Read the model definition and answer for the solid it produces. Units are mm, in the model's axes. A direction names the side the tool comes from. Give positions to 0.01 mm unless a question says otherwise; leave off trailing zeros. Write each loop counter-clockwise with the first axis right and the second up, starting at its lowest first coordinate (ties: lowest second). Pieces come first, ordered by that corner, then holes. Notation, with made-up numbers: (21.25, 79.5) - (31.25, 79.5) arc R30 cw to (31.25, 114.5) - close; hole circle Ø10 at (10, 86). An arc over 180 degrees is marked (long way). Answer as a JSON object with one key per item and string values. Group by question number.
```python
from build123d import *

# Parameters (mm, degrees)
SKETCH1_W           = 95
SKETCH1_H           = 50
BOSS_EXTRUDE1_DEPTH = 5
SKETCH2_W           = 14.5
SKETCH2_H           = 6
BOSS_EXTRUDE2_DEPTH = 32
SKETCH4_R           = 2.75
CUT_EXTRUDE1_DEPTH  = 6
SKETCH6_R           = 2.7
CUT_EXTRUDE2_DEPTH  = 6
BOSS_EXTRUDE5_DEPTH = 32
SKETCH11_R          = 4
CUT_EXTRUDE3_DEPTH  = 6


with BuildPart() as part:
    # Sketch1 → Boss-Extrude1 (new body)
    with BuildSketch(Plane(origin=(0, 0, 0), x_dir=(1, 0, 0), z_dir=(0, 1, 0))):
        Rectangle(SKETCH1_W, SKETCH1_H)
    extrude(amount=BOSS_EXTRUDE1_DEPTH)

    # Sketch2 → Boss-Extrude2 (add)
    with BuildSketch(Plane(origin=(0, 5, 0), x_dir=(1, 0, 0), z_dir=(0, 1, 0))):
        with Locations((-40.25, 22)):
            Rectangle(SKETCH2_W, SKETCH2_H)
        with Locations((40.25, 22)):
            Rectangle(SKETCH2_W, SKETCH2_H)
    extrude(amount=BOSS_EXTRUDE2_DEPTH)

    # Sketch4 → Cut-Extrude1 (cut)
    with BuildSketch(Plane(origin=(0, 0, -25), x_dir=(-1, 0, 0), z_dir=(0, 0, -1))):
        with Locations((37.5, 11.5)):
            Circle(SKETCH4_R)
        with Locations((37.5, 28.5)):
            Circle(SKETCH4_R)
        with Locations(Location((-37.5, 28.5, 0), (0, 0, 180))):
            Circle(SKETCH4_R)
        with Locations(Location((-37.5, 11.5, 0), (0, 0, 180))):
            Circle(SKETCH4_R)
    extrude(amount=-CUT_EXTRUDE1_DEPTH, mode=Mode.SUBTRACT)

    # Sketch6 → Cut-Extrude2 (cut)
    with BuildSketch(Plane(origin=(0, 5, 0), x_dir=(1, 0, 0), z_dir=(0, 1, 0))):
        with Locations(Location((-38, 0, 0), (0, 0, 270))):
            Circle(SKETCH6_R)
        with Locations(Location((38, 0, 0), (0, 0, 270))):
            Circle(SKETCH6_R)
    extrude(amount=-CUT_EXTRUDE2_DEPTH, mode=Mode.SUBTRACT)

    # Sketch10 → Boss-Extrude5 (add)
    with BuildSketch(Plane(origin=(0, 5, 0), x_dir=(1, 0, 0), z_dir=(0, 1, 0))):
        Polygon((-47.5, -14), (-47.5, -25), (-43.5, -25), (43.5, -25), (47.5, -25), (47.5, -19), (47.5, 19), (43.5, 19), (43.5, -19), (-43.5, -19), (-43.5, 19), (-47.5, 19), align=None)
    extrude(amount=BOSS_EXTRUDE5_DEPTH)

    # Sketch11 → Cut-Extrude3 (cut)
    with BuildSketch(Plane.XY.offset(25)):
        with Locations((19, 20)):
            Circle(SKETCH11_R)
    extrude(amount=-CUT_EXTRUDE3_DEPTH, mode=Mode.SUBTRACT)


solid = part.part
```
1) Find the intervals of material crossed by line 1 (Y direction, x = 37.5, z = -22.1); line 2 (X direction, y = 18.5, z = -16.5); line 3 (X direction, y = 1, z = 0), in increasing order. Write a range as [from, to].
2) Find section B-B, the plane z = 0. Write down the section's boundary in (x, y), and give its area (3 significant figures).
3) Which of the six approach directions +Z, -Z, +X, -X, +Y, -Y give full straight-line access (tool end or side, diameter ignored) to faces 1 (the cylindrical face through (-34.753, 28.621, -22.042)), 2 (the flat face through (-43.5, 21, 0)), 3 (the flat face through (-33, 21, -22)), 4 (the cylindrical face through (-40.395, 2.535, 1.246))?
4) Find section D-D, the plane z = 9. Write down the section's boundary in (x, y).
5) For a pull along Y with two mould halves and no side action, classify faces 5 (the cylindrical face through (34.753, 11.379, -22.042)), 6 (the flat face through (33, 21, -22)), 7 (the cylindrical face through (-34.753, 11.621, -22.042)), 8 (the flat face through (3, 37, 20)) as released by +Y, released by -Y, zero draft, split by the parting line, or undercut.
6) Find section C-C, the plane y = 20. Write down the section's boundary in (x, z).
7) Find section A-A, the plane x = 19. Write down the section's boundary in (y, z).
8) Flat-ended cylindrical pins translate along their axes: pin 1 Ø5 at (x, z) = (-31.5, 9) entering from +Y; pin 2 Ø5 at (x, y) = (37.5, 11.5) entering from -Z. Find the tip coordinate at first contact, or state that the pin passes through.
Values follow:
{
 "1": {"line 1": "y = [0, 8.75], [14.25, 25.75], [31.25, 37]", "line 2": "x = [-47.5, -43.5], [43.5, 47.5]", "line 3": "x = [-47.5, -40.7], [-35.3, 35.3], [40.7, 47.5]"},
 "2": {"outline": "(-47.5, 0) - (-40.7, 0) - (-40.7, 5) - (-43.5, 5) - (-43.5, 37) - (-47.5, 37) - close; (-35.3, 0) - (35.3, 0) - (35.3, 5) - (-35.3, 5) - close; (40.7, 0) - (47.5, 0) - (47.5, 37) - (43.5, 37) - (43.5, 5) - (40.7, 5) - close", "area": "677 mm2"},
 "3": {"face 1": "-Z", "face 2": "+Y", "face 3": "-Z, +Y", "face 4": "+Y, -Y"},
 "4": {"outline": "(-47.5, 0) - (47.5, 0) - (47.5, 37) - (43.5, 37) - (43.5, 5) - (-43.5, 5) - (-43.5, 37) - (-47.5, 37) - close"},
 "5": {"face 5": "undercut", "face 6": "zero draft", "face 7": "undercut", "face 8": "released by +Y"},
 "6": {"outline": "(-47.5, -25) - (-33, -25) - (-33, -19) - (-43.5, -19) - (-43.5, 19) - (15, 19) - (15, 25) - (-47.5, 25) - close; (23, 19) - (43.5, 19) - (43.5, -19) - (33, -19) - (33, -25) - (47.5, -25) - (47.5, 25) - (23, 25) - close"},
 "7": {"outline": "(0, -25) - (5, -25) - (5, 19) - (16, 19) - (16, 25) - (0, 25) - close; (24, 19) - (37, 19) - (37, 25) - (24, 25) - close"},
 "8": {"pin 1": "stops at y = 5", "pin 2": "stops at z = 19"}
}
